from build123d import *

# Parameters (mm, degrees)
SKETCH1_W           = 12.6968
SKETCH1_H           = 3.175
BOSS_EXTRUDE1_DEPTH = 3.175


with BuildPart() as part:
    # Sketch1 → Boss-Extrude1 (new body)
    with BuildSketch(Plane(origin=(0, 0, 0), x_dir=(1, 0, 0), z_dir=(0, 1, 0))):
        Polygon((-200.0487998, -36.1077), (203.3016, -36.1077), (203.3016, 36.1077), (-200.0487998, 36.1077), (-200.0487998, 38.9255), (-203.3016, 38.9255), (-203.3016, -38.9255), (-200.0487998, -38.9255), align=None)
        with Locations((-157.842857143, -31.142)):
            Rectangle(SKETCH1_W, SKETCH1_H, mode=Mode.SUBTRACT)
        with Locations((184.15, -31.142)):
            Rectangle(SKETCH1_W, SKETCH1_H, mode=Mode.SUBTRACT)
        with Locations((-131.535714286, -31.142)):
            Rectangle(SKETCH1_W, SKETCH1_H, mode=Mode.SUBTRACT)
        with Locations((-105.228571429, -31.142)):
            Rectangle(SKETCH1_W, SKETCH1_H, mode=Mode.SUBTRACT)
        with Locations((157.842857143, -31.142)):
            Rectangle(SKETCH1_W, SKETCH1_H, mode=Mode.SUBTRACT)
        with Locations((131.535714286, -31.142)):
            Rectangle(SKETCH1_W, SKETCH1_H, mode=Mode.SUBTRACT)
        with Locations((105.228571429, -31.142)):
            Rectangle(SKETCH1_W, SKETCH1_H, mode=Mode.SUBTRACT)
        with Locations((78.921428571, -31.142)):
            Rectangle(SKETCH1_W, SKETCH1_H, mode=Mode.SUBTRACT)
        with Locations((52.614285714, -31.142)):
            Rectangle(SKETCH1_W, SKETCH1_H, mode=Mode.SUBTRACT)
        with Locations((26.307142857, -31.142)):
            Rectangle(SKETCH1_W, SKETCH1_H, mode=Mode.SUBTRACT)
        with Locations((0, -31.142)):
            Rectangle(SKETCH1_W, SKETCH1_H, mode=Mode.SUBTRACT)
        with Locations((-26.307142857, -31.142)):
            Rectangle(SKETCH1_W, SKETCH1_H, mode=Mode.SUBTRACT)
        with Locations((-52.614285714, -31.142)):
            Rectangle(SKETCH1_W, SKETCH1_H, mode=Mode.SUBTRACT)
        with Locations((-78.921428571, -31.142)):
            Rectangle(SKETCH1_W, SKETCH1_H, mode=Mode.SUBTRACT)
        with Locations((-184.15, -31.142)):
            Rectangle(SKETCH1_W, SKETCH1_H, mode=Mode.SUBTRACT)
        with Locations((184.15, 31.142)):
            Rectangle(SKETCH1_W, SKETCH1_H, mode=Mode.SUBTRACT)
        with Locations((-157.842857143, 31.142)):
            Rectangle(SKETCH1_W, SKETCH1_H, mode=Mode.SUBTRACT)
        with Locations((-131.535714286, 31.142)):
            Rectangle(SKETCH1_W, SKETCH1_H, mode=Mode.SUBTRACT)
        with Locations((-105.228571429, 31.142)):
            Rectangle(SKETCH1_W, SKETCH1_H, mode=Mode.SUBTRACT)
        with Locations((-78.921428571, 31.142)):
            Rectangle(SKETCH1_W, SKETCH1_H, mode=Mode.SUBTRACT)
        with Locations((-52.614285714, 31.142)):
            Rectangle(SKETCH1_W, SKETCH1_H, mode=Mode.SUBTRACT)
        with Locations((-26.307142857, 31.142)):
            Rectangle(SKETCH1_W, SKETCH1_H, mode=Mode.SUBTRACT)
        with Locations((0, 31.142)):
            Rectangle(SKETCH1_W, SKETCH1_H, mode=Mode.SUBTRACT)
        with Locations((26.307142857, 31.142)):
            Rectangle(SKETCH1_W, SKETCH1_H, mode=Mode.SUBTRACT)
        with Locations((52.614285714, 31.142)):
            Rectangle(SKETCH1_W, SKETCH1_H, mode=Mode.SUBTRACT)
        with Locations((78.921428571, 31.142)):
            Rectangle(SKETCH1_W, SKETCH1_H, mode=Mode.SUBTRACT)
        with Locations((105.228571429, 31.142)):
            Rectangle(SKETCH1_W, SKETCH1_H, mode=Mode.SUBTRACT)
        with Locations((131.535714286, 31.142)):
            Rectangle(SKETCH1_W, SKETCH1_H, mode=Mode.SUBTRACT)
        with Locations((157.842857143, 31.142)):
            Rectangle(SKETCH1_W, SKETCH1_H, mode=Mode.SUBTRACT)
        with Locations((-184.15, 31.142)):
            Rectangle(SKETCH1_W, SKETCH1_H, mode=Mode.SUBTRACT)
    extrude(amount=BOSS_EXTRUDE1_DEPTH)


solid = part.part
The listing builds one solid part. Answer for the finished solid, in the listing's coordinates (mm). Give positions to 0.01 mm unless a question says otherwise; leave off trailing zeros. Write each loop counter-clockwise with the first axis right and the second up, starting at its lowest first coordinate (ties: lowest second). Pieces come first, ordered by that corner, then holes.
1) Given P1, Ø1.6, axis at x = 133.5, y = 1.5, coming from the +Z side, flat-ended and moving along its own axis, determine where the tip first touches the part or whether it passes through.
2) Section C-C (x = 42.5) is taken. Write down the section's boundary in (y, z) (3 decimals).
3) Find the intervals of material crossed by L1, parallel to Z at x = 54.5, y = 2.1; L2, parallel to Z at x = -120.5, y = 2.25, in increasing order.
4) Section A-A (x = 131) is taken. Write down the section's boundary in (y, z) (1 decimal), and give its area (3 significant figures).
5) Section B-B (y = 1.3) is taken. Count the separate pieces of the cut face and the enclosed holes in it, and give its area (3 significant figures).
Response:
1. P1: stops at z = 36.11
2. outline: (0, -36.108) - (3.175, -36.108) - (3.175, 36.108) - (0, 36.108) - close
3. L1: z = -36.11 to -32.73, -29.55 to 29.55, 32.73 to 36.11
3. L2: z = -36.11 to 36.11
4. outline: (0, -36.1) - (3.2, -36.1) - (3.2, -32.7) - (0, -32.7) - close; (0, -29.6) - (3.2, -29.6) - (3.2, 29.6) - (0, 29.6) - close; (0, 32.7) - (3.2, 32.7) - (3.2, 36.1) - (0, 36.1) - close
4. area: 209 mm2
5. separate pieces: 1
5. enclosed holes: 30
5. area: 28,200 mm2
